Model file for the job. Use its own axes, mm. A direction names the side the tool comes from. Round coordinates to 2 decimals unless told otherwise and drop trailing zeros. Loops run counter-clockwise (first coordinate to the right, second up) from the corner with the lowest first, then second, coordinate; pieces in that order, holes last. Notation, with made-up numbers: (3, 29.5) -> (49, 29.5) arc R17 cw to (49, 37.5) -> close; hole circle Ø2 at (66, 82). An arc over 180 degrees is marked (long way). Use a Markdown table: item, result.
from build123d import *

# Parameters (mm, degrees)
F1_DEPTH = 5.715
F2_SIZE  = 1.778


with BuildPart() as f1:
    # F0 (on Right) → F1 (new body, symmetric)
    with BuildSketch(Plane.YZ):
        with BuildLine():
            Line((0, -19.05), (0, 0))
            Line((0, 0), (0, 19.05))
            Line((0, 19.05), (7.39775, 19.05))
            Line((7.39775, 19.05), (7.39775, 14.2875))
            Line((7.39775, 14.2875), (4.85775, 14.2875))
            Line((4.85775, 14.2875), (4.85775, 11.1125))
            Line((4.85775, 11.1125), (10.57275, 11.1125))
            Line((10.57275, 11.1125), (10.57275, 18.415))
            ThreePointArc((10.57275, 18.415), (9.456827, 21.109077), (6.76275, 22.225))
            Line((6.76275, 22.225), (0.635, 22.225))
            ThreePointArc((0.635, 22.225), (-2.059077, 21.109077), (-3.175, 18.415))
            Line((-3.175, 18.415), (-3.175, 0))
            Line((-3.175, 0), (-3.175, -18.415))
            ThreePointArc((-3.175, -18.415), (-2.059077, -21.109077), (0.635, -22.225))
            Line((0.635, -22.225), (6.76275, -22.225))
            ThreePointArc((6.76275, -22.225), (9.456827, -21.109077), (10.57275, -18.415))
            Line((10.57275, -18.415), (10.57275, -11.1125))
            Line((10.57275, -11.1125), (4.85775, -11.1125))
            Line((4.85775, -11.1125), (4.85775, -14.2875))
            Line((4.85775, -14.2875), (7.39775, -14.2875))
            Line((7.39775, -14.2875), (7.39775, -19.05))
            Line((7.39775, -19.05), (0, -19.05))
        make_face()
    extrude(amount=F1_DEPTH, both=True)

    # F2
    f2_edges = [f1.edges().sort_by_distance(p)[0] for p in [
        (-5.715, 3.698875, -19.05),
        (-5.715, 0, 0),
        (-5.715, 3.698875, 19.05),
    ]]
    chamfer(f2_edges, length=F2_SIZE)


solid = f1.part
Q1. Band-saw the part on C-C, the plane y = 6.25. Give the number of separate pieces and of enclosed holes in the cut face, plus the area to 3 significant figures.
Results list:
| item | result |
|---|---|
| separate pieces | 4 |
| enclosed holes | 0 |
| area | 142 mm² |
Q2. Band-saw the part on A-A, the plane y = 4. Give the cut face in (x, z) (3 decimals).
Results list:
| item | result |
|---|---|
| outline | (-5.715, -22.225) -> (5.715, -22.225) -> (5.715, -19.05) -> (-3.937, -19.05) -> (-5.715, -20.828) -> close; (-5.715, 20.828) -> (-3.937, 19.05) -> (5.715, 19.05) -> (5.715, 22.225) -> (-5.715, 22.225) -> close |
Q3. Tool access for faces 4 (the face through (0, 8, -11.112)), 5 (the face through (5.715, -1, 0)), 6 (the face through (-4.838, 2.746, 19.951)), 7 (the face through (1, 0, 0)): list every direction of +Z, -Z, +X, -X, +Y, -Y with a clear straight run to the whole face (end or side of a thin tool).
Results list:
| item | result |
|---|---|
| face 4 | +X, -X, +Y |
| face 5 | +Z, -Z, +X, +Y, -Y |
| face 6 | -X |
| face 7 | +X, -X |
Q4. Drill centre lines: L1, parallel to Z at x = -3.25, y = 4.25 (3 decimals); L2, parallel to Y at x = 3.25, z = 18 (3 decimals); L3, parallel to Y at x = 0.75, z = 12 (3 decimals). Where is each one in solid material? Low to high. Write a range as from..to.
Results list:
| item | result |
|---|---|
| L1 | z = -22.225..-19.05, 19.05..22.225 |
| L2 | y = -3.175..0, 7.398..10.573 |
| L3 | y = -3.175..0, 4.858..10.573 |
Q5. Pull direction Y, two halves, no side cores. Call faces 1 (the face through (0, 8, 11.112)), 2 (the face through (0, 6, 14.288)), 3 (the face through (0, -3.175, 0)): released by +Y, released by -Y, zero draft, split by the parting line, or undercut.
Results list:
| item | result |
|---|---|
| face 1 | zero draft |
| face 2 | undercut |
| face 3 | released by -Y |
Q6. Flat gauge pins, fed straight in: pin 1 (1 mm diameter, centred on x = 4.5, y = 7.5, fed in from +Z); pin 2 (3 mm diameter, centred on x = -2, y = -1.5, fed in from -Z). Where does each tip first touch, or does it go through?
Results list:
| item | result |
|---|---|
| pin 1 | stops at z = 22.22 |
| pin 2 | stops at z = -22.17 |
Q7. Band-saw the part on B-B, the plane z = 13. Give the cut face in (x, y) (3 decimals), plus the area to 3 significant figures.
Results list:
| item | result |
|---|---|
| outline | (-5.715, -3.175) -> (5.715, -3.175) -> (5.715, 0) -> (-3.937, 0) -> (-5.715, -1.778) -> close; (-5.715, 4.858) -> (5.715, 4.858) -> (5.715, 10.573) -> (-5.715, 10.573) -> close |
| area | 100 mm² |
